Job drawing, mm, ordinate dimensions from the low corner. One solid piece. A direction names the side the tool comes from. Give positions to 0.01 mm unless a question says otherwise; leave off trailing zeros. Write each loop counter-clockwise with the first axis right and the second up, starting at its lowest first coordinate (ties: lowest second). Pieces come first, ordered by that corner, then holes. Notation, with made-up numbers: M -1.75,8.25 L 17.25,8.25 A17 ccw 17.25,27.25 Z; hole C 80.5,62 d3. An arc over 180 degrees is marked long. Use a Markdown table: item, result.
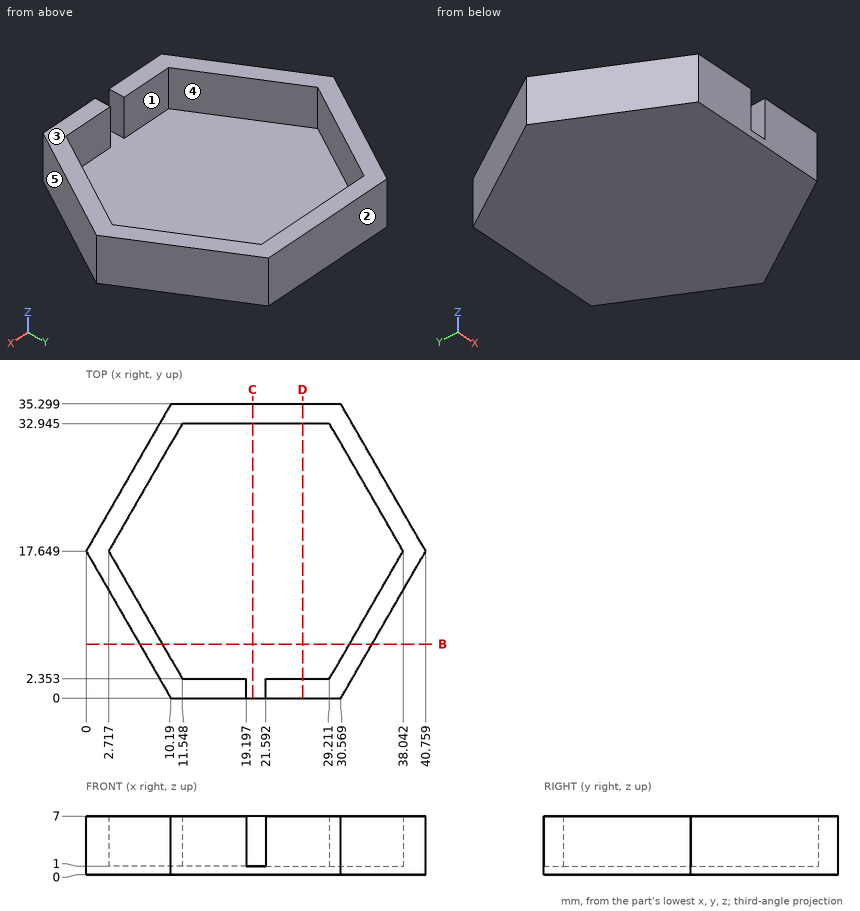
1. Cut at B-B, the plane y = 6.5. Give the cut face in (x, z) (1 decimal).
Findings below:
| item | result |
|---|---|
| outline | M 6.4,0 L 34.3,0 L 34.3,7 L 31.6,7 L 31.6,1 L 9.2,1 L 9.2,7 L 6.4,7 Z |
2. Cut at C-C, the plane x = 20. Give the cut face in (y, z) (1 decimal).
Findings below:
| item | result |
|---|---|
| outline | M 0,0 L 35.3,0 L 35.3,7 L 32.9,7 L 32.9,1 L 0,1 Z |
3. Drop flat-ended pins along their axis: P1, Ø3, axis at y = 8, z = 4, coming from the +X side (1 decimal); P2, Ø10, axis at x = 22.5, y = 17.5, coming from the +Z side; P3, Ø1.2, axis at y = 1.5, z = 3.5, coming from the +X side. Give the stop position or say it passes through.
Findings below:
| item | result |
|---|---|
| P1 | x = 36.1 |
| P2 | z = 1 |
| P3 | x = 31.78 |
4. Drill centre lines: L1, parallel to Y at x = 16.5, z = 3 (1 decimal); L2, parallel to Z at x = 11, y = 15.5; L3, parallel to X at y = 31.5, z = 6 (1 decimal). Where is each one in solid material? Low to high.
Findings below:
| item | result |
|---|---|
| L1 | 0 to 2.4, 32.9 to 35.3 |
| L2 | 0 to 1 |
| L3 | 8 to 10.7, 30 to 32.8 |
5. Cut at D-D, the plane x = 26. Give the cut face in (y, z) (1 decimal).
Findings below:
| item | result |
|---|---|
| outline | M 0,0 L 35.3,0 L 35.3,7 L 32.9,7 L 32.9,1 L 2.4,1 L 2.4,7 L 0,7 Z |
6. Tool access for the marked faces 1 and 2: list every direction of +Z, -Z, +X, -X, +Y, -Y with a clear straight run to the whole face (end or side of a thin tool).
Findings below:
| item | result |
|---|---|
| face 1 | +Z |
| face 2 | +Z, -Z, +X, -X, +Y |
7. Two-plate mould, pull along Y, no slides. Class the marked faces 3, 4 and 5: released by +Y, released by -Y, zero draft, split by the parting line, or undercut.
Findings below:
| item | result |
|---|---|
| face 3 | zero draft |
| face 4 | undercut |
| face 5 | released by -Y |
